Part print with two shaded views. Sizes in mm from the minimum x, y, z corner. A direction names the side the tool comes from. Round coordinates to 2 decimals unless told otherwise and drop trailing zeros. Order: outer loops, then holes, each group sorted by start corner. A loop starts at its lowest first (then second) coordinate and runs counter-clockwise, first axis right, second up. Notation, with made-up numbers: M -32,89.5 L 24,89.5 A28 cw 24,128.5 Z; hole C 75,47.25 d10. An arc over 180 degrees is marked long. Return JSON: item names as keys, results as strings. Group by question number.
Item 1: Slice it at C-C on y = 3.5. Write the cut outline in (x, z).
Item 2: Slice it at B-B on x = 9.25. Write the cut outline in (y, z).
Item 3: Pin check, flat tips, straight feed: pin 1 Ø3 at (x, z) = (18, 2.5) entering from +Y; pin 2 Ø1 at (x, y) = (9, 1) entering from +Z; pin 3 Ø6 at (x, z) = (6.5, 12) entering from -Y. Stop position of each tip, or through.
Item 4: Probe line 1 along X through (y, z) = (2.7, 2.5); line 2 along Z through (x, y) = (15.5, 1.25); line 3 along X through (y, z) = (2.4, 10). List the from-to ranges inside material, lowest first.
Item 5: Slice it at D-D on z = 4.75. Write the cut outline in (x, y), then the cut area to 3 significant figures.
Item 6: Slice it at A-A on y = 1.6. Write the cut outline in (x, z), then the cut area to 3 significant figures.
Item 7: Which spindle directions (+Z, -Z, +X, -X, +Y, -Y) get a long thin tool onto all of the face, cutting with end or side? Do the marked faces 1 and 2. Say none if no direction does.
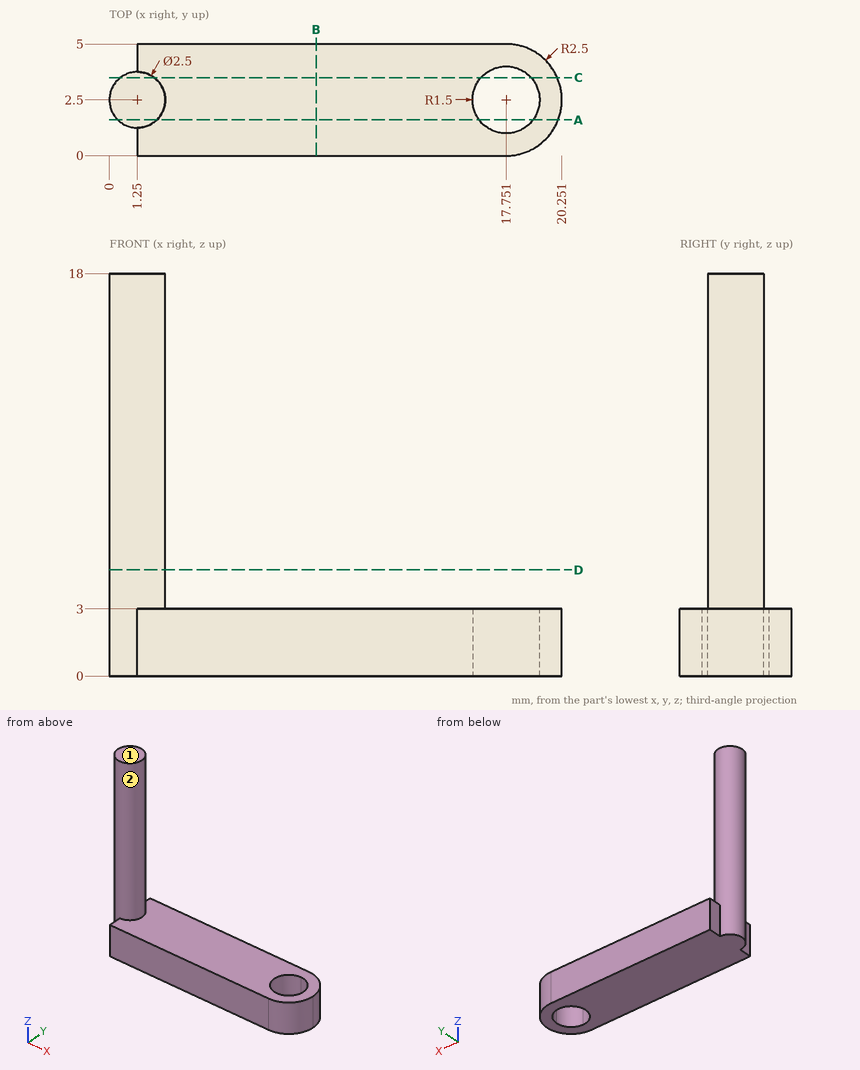
Output values:
{
 "1": {"outline": "M 0.5,0 L 16.63,0 L 16.63,3 L 2,3 L 2,18 L 0.5,18 Z; M 18.87,0 L 20.04,0 L 20.04,3 L 18.87,3 Z"},
 "2": {"outline": "M 0,0 L 5,0 L 5,3 L 0,3 Z"},
 "3": {"pin 1": "y = 5", "pin 2": "z = 3", "pin 3": "through"},
 "4": {"line 1": "0.02 to 16.26, 19.24 to 20.24", "line 2": "0 to 3", "line 3": "0 to 2.5"},
 "5": {"outline": "C 1.25,2.5 d2.5", "area": "4.91 mm²"},
 "6": {"outline": "M 0.38,0 L 16.55,0 L 16.55,3 L 2.12,3 L 2.12,18 L 0.38,18 Z; M 18.95,0 L 20.08,0 L 20.08,3 L 18.95,3 Z", "area": "77.9 mm²"},
 "7": {"face 1": "+Z, +X, -X, +Y, -Y", "face 2": "+Z"}
}
